Autodesk Inventor part; units mm, degrees
ref_plane "Work Plane1" through (-6, 0, 0) normal (1, 0, 0) x (0, 0, -1)
ref_plane "Work Plane2" through (5, 0, 0) normal (0, 0, -1) x (1, 0, 0)
ref_plane "YZ Plane" through (0, 0, 0) normal (1, 0, 0) x (0, 1, 0)
sketch "草图1" plane through (0, 0, 0) normal (0, 0, 1) x (1, 0, 0)
  line L0 (-9.6282, 0) -> (13.485, 0)
  line L1 (0, -1.0134) -> (0, 6.0805)
  line L2 (-6, 0) -> (10, 0)
  line L3 (10, 0) -> (10, 4)
  line L4 (10, 4) -> (0, 4)
  line L5 (0, 4) -> (0, 4.98)
  line L6 (0, 4.98) -> (-4.6718, 4.98)
  arc A0 (-4.6718, 4.98) -> (-6, 0) centre (4, 0) ccw
  line L7 (0, 4) -> (2, 4)
  line L8 (2, 3.1) -> (0, 3.1) construction
  line L9 (0, 4.35) -> (0, 4)
  line L10 (0, 4.35) -> (0, 3.1) construction
  line L11 (2, 4.35) -> (2, 3.1) construction
  arc A1 (10, 0) -> (9.2614, 4) centre (-1.2, 0) ccw
  line L12 (2, 4) -> (2, 3.5)
  line L13 (1.6, 3.1) -> (0.4, 3.1)
  line L14 (0, 3.5) -> (0, 4)
  arc A2 (0, 3.5) -> (0.4, 3.1) centre (0.4, 3.5) ccw
  arc A3 (1.6, 3.1) -> (2, 3.5) centre (1.6, 3.5) ccw
  dimension "d0" = 10
  dimension "d1" = 6
  dimension "d2" = 8
  dimension "d3" = 9.96
  dimension "d4" = 10
  dimension "d10" = 6.2
  dimension "d11" = 2
  dimension "d12" = 11.2
  dimension "d23" = 0.4
revolve "轴承体" add sketch "草图1" angle 360 about axis through (-6, 0, 0) along (1, 0, 0)
ref_plane "Work Plane1" through (-6, 0, 0) normal (1, 0, 0) x (0, 0, -1)
sketch "草图2" plane through (-6, 0, 0) normal (1, 0, 0) x (0, 0, -1)
  circle A0 centre (0, 0) radius 4.98
  line L0 (0, -6.972) -> (0, 6.972)
  line L1 (6.972, 0) -> (-6.972, 0)
  line L2 (-4.98, 0.75) -> (4.98, 0.75)
  line L3 (4.98, 0.75) -> (4.98, -0.75)
  line L4 (4.98, -0.75) -> (-4.98, -0.75)
  line L5 (-4.98, -0.75) -> (-4.98, 0.75)
  line L6 (-4.98, 0) -> (4.98, 0) construction
  line L7 (0, 0.75) -> (0, -0.75) construction
  dimension "d7" = 1.5
extrude "开槽" cut sketch "草图2" along normal blind 2.5 contours L1 L0 L2 A0 | L3 L4 A0 | A0 L4 L0 L1 | A0 L2 L3 | L1 A0 L2 L0 | L0 L4 A0 L1 | L5 L2 A0 | A0 L4 L5
thread "螺纹"
revolve "圆角1" cut sketch "草图1" angle 360 about axis through (-6, 0, 0) along (1, 0, 0) contours A1 L4 L3
revolve "沟槽1" cut sketch "草图1" angle 360 about axis through (-6, 0, 0) along (1, 0, 0) contours L1 L4 L12 A3 L13 A2
ref_plane "Work Plane2" through (5, 0, 0) normal (0, 0, -1) x (1, 0, 0)
equation "\"d7\" = SBR"
equation "\"d8\" = STI"
equation "\"d0\" = GEL"
equation "\"d1\" = SHL"
equation "\"d2\" = NND"
equation "\"d3\" = KOD"
equation "\"d4\" = KR"
equation "\"d10\" = GDM"
equation "\"d11\" = GAL"
equation "\"d12\" = 1.4 * NND"
equation "\"d23\" = R1"
equation "\"d13\" = GEL"
equation "\"NND\" = 8"
equation "\"GEL\" = KR"
equation "\"KOD\" = 9.96"
equation "\"STI\" = 2.5"
equation "\"SBR\" = 1.5"
equation "\"GAL\" = 2"
equation "\"KR\" = 10"
equation "\"BDM\" = 9.96"
equation "\"GDM\" = 6.2"
equation "\"SHL\" = KOH"
equation "\"d6\" = -SHL"
equation "\"R1\" = 0.4"
equation "\"GUL\" = 0.61345 * PTC"
equation "\"KOH\" = 6"
equation "\"THREADDIA\" = 8"
equation "\"TOA\" = 30deg"
equation "\"NLG\" = 16"
equation "\"PTC\" = 1.25"
equation "\"RR1\" = 8"
equation "\"GD1\" = THREADDIA - 1.2269 * PTC"
properties part number "螺钉 GB 831 M8 x 6" material "钢，软"
Source: CAD feature listing. Evaluate the final solid. Frame: model axes, mm. A direction names the side the tool comes from. Give positions to 0.01 mm unless a question says otherwise; leave off trailing zeros. Loops run counter-clockwise (first coordinate to the right, second up) from the corner with the lowest first, then second, coordinate; pieces in that order, holes last. Notation, with made-up numbers: (16.5, 42.25) - (66.5, 42.25) arc R15 ccw to (66.5, 59.25) - close; hole circle Ø8 at (3, -24). An arc over 180 degrees is marked (long way). Use CSV: the item, a comma, the result in double quotes.
1) Line query: line 1 (Y direction, x = -4.5, z = -3); line 2 (Z direction, x = 6.5, y = 0); line 3 (Y direction, x = -4.75, z = 0.25). Output: solid intervals per line, ascending.
Worked out:
line 1,"y = -3.97 to -0.75, 0.75 to 3.97"
line 2,"z = -4 to 4"
line 3,"y = -4.83 to -0.75, 0.75 to 4.83"
2) Cut plane B-B (x = 3). Output: boundary loops of the cut face in (y, z).
Worked out:
outline,"circle Ø8 at (0, 0)"
3) Set-up query: faces 1 (the cylindrical face through (0.99, 1.43, 2.75)), 2 (the flat face through (-4, 0.75, 0)), 3 (the cylindrical face through (5.58, -0.867, 3.905)), 4 (the cylindrical face through (-2.37, -1.08, 4.86)). Return all of +Z, -Z, +X, -X, +Y, -Y with unobstructed straight access to the full face (end or side cutting, diameter ignored); none if empty.
Worked out:
face 1,"none"
face 2,"+Z, -Z, -X"
face 3,"+X"
face 4,"+X, -X"
4) Mould query, pull axis X, two halves, no side actions, for faces 5 (the flat face through (-3.5, 0, 0)), 6 (the flat face through (0, 2.1, -3.3)), 7 (the flat face through (-4, -0.75, 0)). Classes: +X half, -X half, draft (parallel to the pull), parting line (faces both ways), or undercut.
Worked out:
face 5,"-X half"
face 6,"undercut"
face 7,"draft"
5) Cut plane A-A (x = -0.5). Output: boundary loops of the cut face in (y, z), and give its area (3 significant figures).
Worked out:
outline,"circle Ø9.96 at (0, 0)"
area,"77.9 mm^2"
6) Pin query (flat end, axial travel): P1, Ø3, axis at y = -1.5, z = -0.5, coming from the +X side; P2, Ø1, axis at y = 3, z = -3.5, coming from the +X side; P3, Ø3, axis at y = 2, z = -2.5, coming from the +X side; P4, Ø5, axis at x = 7.5, z = 1, coming from the -Y side. Return the tip coordinate at first contact, or that it passes through.
Worked out:
P1,"stops at x = 10"
P2,"stops at x = 0"
P3,"stops at x = 9.87"
P4,"stops at y = -4"
